Model file for the job. Use its own axes, mm. A direction names the side the tool comes from. Round coordinates to 2 decimals unless told otherwise and drop trailing zeros. Loops run counter-clockwise (first coordinate to the right, second up) from the corner with the lowest first, then second, coordinate; pieces in that order, holes last. Notation, with made-up numbers: (3.5, 38) - (47.5, 38) arc R10 cw to (47.5, 52) - close; hole circle Ø10 at (56.5, -11). An arc over 180 degrees is marked (long way). Answer as a JSON object with one key per item and string values.
from build123d import *

# Parameters (mm, degrees)
SKETCH_R     = 2
PAD_DEPTH    = 4
SKETCH001_W  = 15
SKETCH001_H  = 4
POCKET_DEPTH = 5


with BuildPart() as part:
    # Sketch → Pad (new body)
    with BuildSketch(Plane.XZ):
        with BuildLine():
            Line((0, 25), (0, 0))
            Line((0, 0), (70, 0))
            Line((70, 25), (70, 0))
            ThreePointArc((70, 25), (61.213203, 46.213203), (40, 55))
            Line((40, 51), (40, 55))
            Line((30, 51), (40, 51))
            Line((30, 55), (30, 51))
            ThreePointArc((30, 55), (8.786797, 46.213203), (0, 25))
        make_face()
        with Locations((35, 12)):
            Circle(SKETCH_R, mode=Mode.SUBTRACT)
    extrude(amount=PAD_DEPTH)

    # Sketch001 (on Face11 of Pad) → Pocket (cut)
    with BuildSketch(Plane.XZ.offset(4)):
        with Locations((7.5, 2)):
            Rectangle(SKETCH001_W, SKETCH001_H)
        with Locations((62.5, 2)):
            Rectangle(SKETCH001_W, SKETCH001_H)
    extrude(amount=-POCKET_DEPTH, mode=Mode.SUBTRACT)


solid = part.part
1) Slice it at C-C on y = -1.25. List the corners of the cut face in (x, z).
Values follow:
{"outline": "(0, 4) - (15, 4) - (15, 0) - (55, 0) - (55, 4) - (70, 4) - (70, 25) arc R30 ccw to (40, 55) - (40, 51) - (30, 51) - (30, 55) arc R30 ccw to (0, 25) - close; hole circle Ø4 at (35, 12)"}
2) Drop flat-ended pins along their axis: P1, Ø2, axis at y = -2.5, z = 1.5, coming from the +X side; P2, Ø1.2, axis at x = 8.5, y = -2.5, coming from the -Z side; P3, Ø3, axis at x = 35, z = 12, coming from the +Y side; P4, Ø1.5, axis at y = -3.5, z = 37.5, coming from the +X side. Give the stop position or say it passes through.
Values follow:
{"P1": "x = 55", "P2": "z = 4", "P3": "through", "P4": "x = 67.6"}
3) Slice it at D-D on x = 11.5. List the corners of the cut face in (y, z), then the cut area to 3 significant figures.
Values follow:
{"outline": "(-4, 4) - (0, 4) - (0, 48.62) - (-4, 48.62) - close", "area": "178 mm²"}
4) Tool access for faces 1 (the flat face through (62, -2, 4)), 2 (the flat face through (30, -2, 53)), 3 (the flat face through (7, -2, 4)): list every direction of +Z, -Z, +X, -X, +Y, -Y with a clear straight run to the whole face (end or side of a thin tool).
Values follow:
{"face 1": "-Z, +X, +Y, -Y", "face 2": "+Z, +Y, -Y", "face 3": "-Z, -X, +Y, -Y"}
5) Two-plate mould, pull along X, no slides. Class faces 4 (the flat face through (35, -4, 28)), 5 (the flat face through (40, -2, 53)), 6 (the flat face through (15, -2, 2)), 7 (the flat face through (35, -2, 51)): pulls with the +X half, pulls with the -X half, needs draft (parallel to the pull), parting line crosses it, or undercut.
Values follow:
{"face 4": "needs draft", "face 5": "undercut", "face 6": "pulls with the -X half", "face 7": "undercut"}
6) Probe probe 1 along Z at (x, y) = (35, -1.3); probe 2 along Z at (x, y) = (24, -3.6); probe 3 along Z at (x, y) = (47, -0.25). List the from-to ranges inside material, lowest first.
Values follow:
{"probe 1": "0 to 10, 14 to 51", "probe 2": "0 to 54.39", "probe 3": "0 to 54.17"}
7) Slice it at A-A on z = 12. List the corners of the cut face in (x, y), then the cut area to 3 significant figures.
Values follow:
{"outline": "(0, -4) - (33, -4) - (33, 0) - (0, 0) - close; (37, -4) - (70, -4) - (70, 0) - (37, 0) - close", "area": "264 mm²"}
8) Slice it at B-B on x = 35. List the corners of the cut face in (y, z), then the cut area to 3 significant figures.
Values follow:
{"outline": "(-4, 0) - (0, 0) - (0, 10) - (-4, 10) - close; (-4, 14) - (0, 14) - (0, 51) - (-4, 51) - close", "area": "188 mm²"}
